from build123d import *

# Parameters (mm, degrees)
BOSS_EXTRUDE1_DEPTH            = 2.5
F_2_5MM_DOWEL_HOLE1_AT_2_COUNT = 2
F_2_5MM_DOWEL_HOLE1_AT_2_PITCH = 43.617065155


with BuildPart() as part:
    # Sketch1 → Boss-Extrude1 (new, symmetric)
    with BuildSketch(Plane(origin=(0, 0, 0), x_dir=(0, 0, -1), z_dir=(1, 0, 0))):
        Polygon((0, 65), (0, 0), (65, 0), (65, 10), (10, 65), align=None)
    extrude(amount=BOSS_EXTRUDE1_DEPTH, both=True)

    # Sketch3 → Ø2.5mm Dowel Hole1 (revolve, cut)
    with BuildSketch(Plane(origin=(2.5, 47.617660414, -16.775737868), x_dir=(0, 0, -1), z_dir=(0, 1, 0))):
        Polygon((0, 0), (0, 5), (1.275, 5), (1.25, 4.975), (1.25, 0), align=None)
    f_2_5mm_dowel_hole1 = revolve(axis=Axis((8.85, 47.617660414, -16.775737868), (-1, 0, 0)), mode=Mode.SUBTRACT)

    # Ø2.5mm Dowel Hole1 at 2: Ø2.5mm Dowel Hole1 ×2
    with Locations(*[Vector(0, -0.7071067811865474, -0.7071067811865477) * (i * F_2_5MM_DOWEL_HOLE1_AT_2_PITCH) for i in range(1, F_2_5MM_DOWEL_HOLE1_AT_2_COUNT)]):
        add(f_2_5mm_dowel_hole1, mode=Mode.SUBTRACT)


solid = part.part
Build history of the part. All positions in model axes, mm. Give positions to 0.01 mm unless a question says otherwise; leave off trailing zeros. Order: outer loops, then holes, each group sorted by start corner. A loop starts at its lowest first (then second) coordinate and runs counter-clockwise, first axis right, second up. Notation, with made-up numbers: M -5,13 L 13,13 A21 cw 13,20 Z; hole C -15,7 d6. An arc over 180 degrees is marked long. Use one line per item in the form item = value.
Q1. Slice it at A-A, the plane x = 0.6. Write the cut outline in (y, z), and give its area (3 significant figures).
Conclusion:
outline = M 0,-65 L 10,-65 L 65,-10 L 65,0 L 0,0 Z; hole C 16.78,-47.62 d2.5; hole C 47.62,-16.78 d2.5
area = 2,700 mm2
Q2. Wall check: probe 1 along Z at (x, y) = (1.2, 17.5); probe 2 along Y at (x, z) = (2, -16.5); probe 3 along Y at (x, z) = (1.4, -48.5). Give the ranges that are in metal, low to high.
Conclusion:
probe_1 = -57.5 to -48.64, -46.6 to 0
probe_2 = 0 to 46.4, 48.84 to 58.5
probe_3 = 0 to 15.89, 17.66 to 26.5
Q3. Slice it at C-C, the plane y = 32.5. Write the cut outline in (x, z), and give its area (4 significant figures).
Conclusion:
outline = M -2.5,-42.5 L 2.5,-42.5 L 2.5,0 L -2.5,0 Z
area = 212.5 mm2
Q4. Pull direction Z, two halves, no side cores. Call faces 1 (the flat face through (0, 33, 0)), 2 (the cylindrical face through (0.05, 16.4, -48.81)), 3 (the flat face through (0, 5, -65)), 4 (the cylindrical face through (0.05, 48.1, -17.93)): released by +Z, released by -Z, zero draft, split by the parting line, or undercut.
Conclusion:
face_1 = released by +Z
face_2 = undercut
face_3 = released by -Z
face_4 = undercut
Q5. Pin check, flat tips, straight feed: P1, Ø8, axis at y = 35, z = -48.5, coming from the -X side; P2, Ø12, axis at y = 29.5, z = -46, coming from the +X side; P3, Ø1, axis at x = 2, y = 42, coming from the -Z side. Stop position of each tip, or through.
Conclusion:
P1 = through
P2 = 2.5
P3 = -33.5
Q6. Slice it at B-B, the plane z = -52.5. Write the cut outline in (x, y), and give its area (4 significant figures).
Conclusion:
outline = M -2.5,0 L 2.5,0 L 2.5,22.5 L -2.5,22.5 Z
area = 112.5 mm2
